Design review of the part shown in the three views and the two pictorial views. Dimensions are in mm from the part's minimum x, y and z. Give positions to 0.01 mm unless a question says otherwise; leave off trailing zeros. Order: outer loops, then holes, each group sorted by start corner. A loop starts at its lowest first (then second) coordinate and runs counter-clockwise, first axis right, second up.
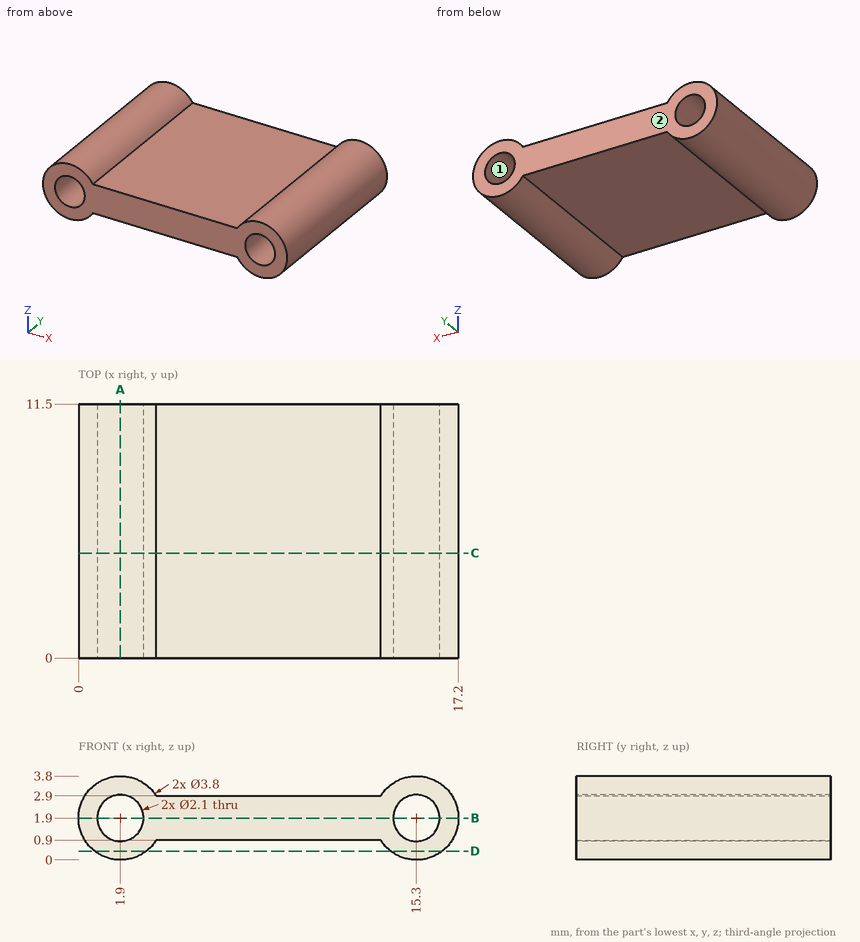
1) To check wall thickness, follow line 1 (X direction, y = 7.25, z = 1.95); line 2 (X direction, y = 8.5, z = 1.45); line 3 (Z direction, x = 15.3, y = 5.75). State the ranges of each line that lie inside material, in increasing order.
Answer sheet:
line 1: x = 0 to 0.85, 2.95 to 14.25, 16.35 to 17.2
line 2: x = 0.05 to 0.95, 2.85 to 14.35, 16.25 to 17.15
line 3: z = 0 to 0.85, 2.95 to 3.8
2) We need section D-D on z = 0.4. Give the boundary of the cut face in (x, y).
Answer sheet:
outline: (0.73, 0) - (3.07, 0) - (3.07, 11.5) - (0.73, 11.5) - close; (14.13, 0) - (16.47, 0) - (16.47, 11.5) - (14.13, 11.5) - close
3) We need section A-A on x = 1.9. Give the boundary of the cut face in (y, z), then the cut area to 4 significant figures.
Answer sheet:
outline: (0, 0) - (11.5, 0) - (11.5, 0.85) - (0, 0.85) - close; (0, 2.95) - (11.5, 2.95) - (11.5, 3.8) - (0, 3.8) - close
area: 19.55 mm2
4) We need section B-B on z = 1.9. Give the boundary of the cut face in (x, y), then the cut area to 4 significant figures.
Answer sheet:
outline: (0, 0) - (0.85, 0) - (0.85, 11.5) - (0, 11.5) - close; (2.95, 0) - (14.25, 0) - (14.25, 11.5) - (2.95, 11.5) - close; (16.35, 0) - (17.2, 0) - (17.2, 11.5) - (16.35, 11.5) - close
area: 149.5 mm2
5) Draft analysis for pull direction X (two halves, no side actions). For the marked faces 1 and 2, state which applies: +X half, -X half, draft (parallel to the pull), parting line (faces both ways), or undercut.
Answer sheet:
face 1: undercut
face 2: draft
6) Clearance check with flat-ended pins moving along their axes: pin 1 (1 mm diameter, centred on x = 2, z = 2, fed in from -Y); pin 2 (4 mm diameter, centred on x = 13, y = 3, fed in from -Z); pin 3 (3 mm diameter, centred on x = 10, y = 8, fed in from -Z). State where each tip first meets the part, or that it passes through.
Answer sheet:
pin 1: passes through
pin 2: stops at z = 0.02
pin 3: stops at z = 0.9
7) We need section C-C on y = 4.75. Give the boundary of the cut face in (x, z), then the cut area to 3 significant figures.
Answer sheet:
outline: (3.52, 0.9) - (13.68, 0.9) arc R1.9 ccw (long way) to (13.68, 2.9) - (3.52, 2.9) arc R1.9 ccw (long way) to start; hole circle Ø2.1 at (1.9, 1.9); hole circle Ø2.1 at (15.3, 1.9)
area: 35.3 mm2
